Could you check a few things on this model? Use its own coordinates, in mm. Face numbers are marked on the shaded views. A direction names the side the tool comes from. Round coordinates to 2 decimals unless told otherwise and drop trailing zeros. Write each loop counter-clockwise with the first axis right and the second up, starting at its lowest first coordinate (ties: lowest second). Pieces come first, ordered by that corner, then holes. Notation, with made-up numbers: M 78,-16 L 136,-16 A16 cw 136,-11 Z; hole C 20,20.5 d8. An arc over 180 degrees is marked long. One line per item, written item: value. Start each with the question number.
(1) I want a section at D-D on z = -16. Please give me the cut outline in (x, y).
(2) I want a section at A-A on y = -12.7. Please give me the cut outline in (x, z), and give its area (3 significant figures).
(3) I want a section at C-C on y = -7. Please give me the cut outline in (x, z), and give its area (3 significant figures).
(4) Thinking about a two-plate mould opening in Y: for the marked faces 3, 4, 5 and 6, which applies, released by +Y, released by -Y, zero draft, split by the parting line, or undercut?
(5) I'm going to push flat-ended pins straight in: pin 1 Ø4 at (x, z) = (24.5, 39) entering from -Y; pin 2 Ø4 at (x, y) = (23.5, -29) entering from +Z; pin 3 Ø1 at (x, y) = (31, -26) entering from -Z. Where does each tip first touch, or does it pass through?
(6) Which directions (+Z, -Z, +X, -X, +Y, -Y) give clear straight access to the entire face, cutting with the end or side of a thin tool? Please do the marked faces 1 and 2.
(7) I want a section at B-B on z = 20.5. Please give me the cut outline in (x, y).
(8) If I drill on L1, parallel to Z at x = 27, y = -12.7; L2, parallel to Y at x = 30, z = 14; L3, parallel to Y at x = 15.5, z = -35, over which ranges is the centre line in solid material (lowest first)?
```python
from build123d import *

# Parameters (mm, degrees)
F0_W     = 50.8
F0_H     = 101.6
F1_DEPTH = 25.4
F2_R     = 9.525
F3_DEPTH = 50.8
F4_SIZE  = 5.08
F7_DEPTH = 50.8
F8_R     = 5.08


# Not quite as in the source:
# - a feature of the source that left no trace in its solid (it failed there, or was rolled back) is left out


with BuildPart() as f1:
    # F0 (on Front) → F1 (new body)
    with BuildSketch(Plane.XZ):
        with Locations((20.7021635301, -10.4186603248)):
            Rectangle(F0_W, F0_H)
    extrude(amount=F1_DEPTH)

    # F2 (on face) → F3 (cut)
    with BuildSketch(Plane.YZ.offset(46.1021635301)):
        with Locations((-12.7, 14.9813396752)):
            Circle(F2_R)
        with Locations((-12.7, -35.8186603248)):
            Circle(F2_R)
    extrude(amount=-F3_DEPTH, mode=Mode.SUBTRACT)

    # F4
    f4_edges = [f1.edges().sort_by_distance(p)[0] for p in [
        (-4.697836, -12.7, -61.21866),
        (46.102164, -12.7, -61.21866),
        (20.702164, 0, -61.21866),
        (20.702164, -25.4, -61.21866),
    ]]
    chamfer(f4_edges, length=F4_SIZE)

    # F6 (on face) → F7 (join)
    with BuildSketch(Plane(origin=(-4.6978364699, 0, 0), x_dir=(0, -1, 0), z_dir=(-1, 0, 0))):
        Polygon((50.8, 35.3013396752), (25.4, 35.3013396752), (25.4, -56.1386603248), align=None)
    extrude(amount=-F7_DEPTH)

    # F8
    f8_edges = [f1.edges().sort_by_distance(p)[0] for p in [
        (20.702164, -50.8, 35.30134),
        (20.702164, 0, 40.38134),
        (20.702164, -25.4, -56.13866),
        (20.702164, 0, -56.13866),
    ]]
    fillet(f8_edges, radius=F8_R)


solid = f1.part
```
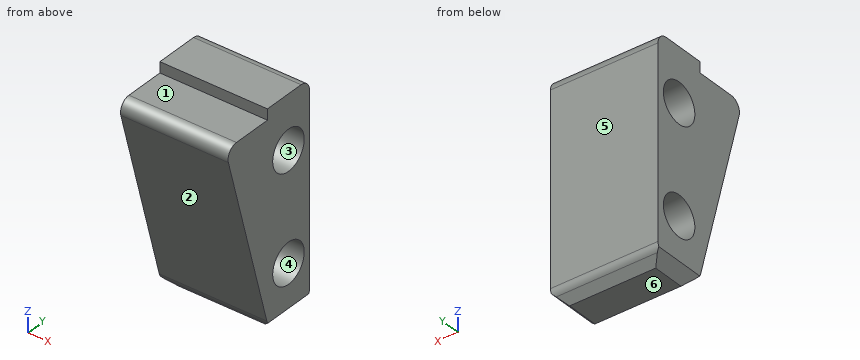
Found:
1. outline: M -4.7,-36.55 L 46.1,-36.55 L 46.1,0 L -4.7,0 Z
2. outline: M -4.7,-56.14 L 0.38,-61.22 L 41.02,-61.22 L 46.1,-56.14 L 46.1,-45.34 L -4.7,-45.34 Z; M -4.7,-26.29 L 46.1,-26.29 L 46.1,5.46 L -4.7,5.46 Z; M -4.7,24.51 L 46.1,24.51 L 46.1,40.38 L -4.7,40.38 Z
2. area: 3,200 mm²
3. outline: M -4.7,-56.14 L 0.38,-61.22 L 41.02,-61.22 L 46.1,-56.14 L 46.1,-43.45 L -4.7,-43.45 Z; M -4.7,-28.19 L 46.1,-28.19 L 46.1,7.35 L -4.7,7.35 Z; M -4.7,22.61 L 46.1,22.61 L 46.1,40.38 L -4.7,40.38 Z
3. area: 3,580 mm²
4. face 3: undercut
4. face 4: undercut
4. face 5: released by +Y
4. face 6: zero draft
5. pin 1: stops at y = -25.4
5. pin 2: stops at z = 35.3
5. pin 3: stops at z = -55.57
6. face 1: +Z, +X, -X, -Y
6. face 2: -Z, +X, -X, -Y
7. outline: M -4.7,-46.69 L 46.1,-46.69 L 46.1,-20.46 L -4.7,-20.46 Z; M -4.7,-4.94 L 46.1,-4.94 L 46.1,0 L -4.7,0 Z
8. L1: z = -61.22 to -45.34, -26.29 to 5.46, 24.51 to 40.38
8. L2: y = -44.88 to -22.17, -3.23 to 0
8. L3: y = -31.27 to -22.19, -3.21 to 0
